from build123d import *

# Parameters (mm, degrees)
F1_DEPTH = 25
F2_R     = 8
F3_DEPTH = 25
F4_SIZE  = 5
F5_R     = 1.75
F6_DEPTH = 25


with BuildPart() as f1:
    # F0 (on Right) → F1 (new body)
    with BuildSketch(Plane.YZ):
        with BuildLine():
            Line((1.7320508076, 42.9015853287), (0, 41.9015853287))
            Line((0, 41.9015853287), (21, 5.5285183697))
            ThreePointArc((21, 5.5285183697), (22.8301270189, 3.6983913508), (25.3301270189, 3.0285183697))
            Line((25.3301270189, 3.0285183697), (72.3301270189, 3.0285183697))
            Line((72.3301270189, 3.0285183697), (72.3301270189, 5.0285183697))
            Line((72.3301270189, 5.0285183697), (25.3301270189, 5.0285183697))
            ThreePointArc((25.3301270189, 5.0285183697), (23.8301270189, 5.4304421584), (22.7320508076, 6.5285183697))
            Line((22.7320508076, 6.5285183697), (1.7320508076, 42.9015853287))
        make_face()
    extrude(amount=F1_DEPTH)

    # F2 (on face) → F3 (cut)
    with BuildSketch(Plane(origin=(0, 19.8759694843, 11.4753963322), x_dir=(-1, 0, 0), z_dir=(0, 0.8660254038, 0.5))):
        with Locations((-12.5, 24.2878373535)):
            Circle(F2_R)
    extrude(amount=-F3_DEPTH, mode=Mode.SUBTRACT)

    # F4
    f4_edges = [f1.edges().sort_by_distance(p)[0] for p in [
        (0, 0.866025, 42.401585),
        (25, 0.866025, 42.401585),
    ]]
    chamfer(f4_edges, length=F4_SIZE)

    # F5 (on face) → F6 (cut)
    with BuildSketch(Plane.XY.offset(5.0285183697)):
        with Locations((12.5, 63.3301270189)):
            Circle(F5_R)
        with Locations((12.5, 48.3301270189)):
            Circle(F5_R)
    extrude(amount=-F6_DEPTH, mode=Mode.SUBTRACT)


solid = f1.part
Build history of the part. All positions in model axes, mm. Round coordinates to 2 decimals unless told otherwise and drop trailing zeros. Loops run counter-clockwise (first coordinate to the right, second up) from the corner with the lowest first, then second, coordinate; pieces in that order, holes last. Notation, with made-up numbers: (12.25, 60) -> (63.25, 60) arc R19 ccw to (63.25, 65) -> close; hole circle Ø11 at (84.25, 65). An arc over 180 degrees is marked (long way). Answer in a Markdown table with one row per item.
Item 1: Saw through at B-B (y = 39). Write the cut outline in (x, z), and give its area (3 significant figures).
Answers below:
| item | result |
|---|---|
| outline | (0, 3.03) -> (25, 3.03) -> (25, 5.03) -> (0, 5.03) -> close |
| area | 50.0 mm² |
Item 2: Saw through at A-A (x = 12.5). Write the cut outline in (y, z).
Answers below:
| item | result |
|---|---|
| outline | (0, 41.9) -> (2, 38.44) -> (3.73, 39.44) -> (1.73, 42.9) -> close; (10, 24.58) -> (21, 5.53) arc R5 ccw to (25.33, 3.03) -> (46.58, 3.03) -> (46.58, 5.03) -> (25.33, 5.03) arc R3 cw to (22.73, 6.53) -> (11.73, 25.58) -> close; (50.08, 3.03) -> (61.58, 3.03) -> (61.58, 5.03) -> (50.08, 5.03) -> close; (65.08, 3.03) -> (72.33, 3.03) -> (72.33, 5.03) -> (65.08, 5.03) -> close |
Item 3: Pin check, flat tips, straight feed: pin 1 (8 mm diameter, centred on x = 11, z = 29.5, fed in from +Y); pin 2 (10 mm diameter, centred on x = 11.5, z = 8.5, fed in from -Y); pin 3 (6 mm diameter, centred on x = 5, z = 14.5, fed in from -Y). Stop position of each tip, or through.
Answers below:
| item | result |
|---|---|
| pin 1 | stops at y = 11.78 |
| pin 2 | stops at y = 16.4 |
| pin 3 | stops at y = 14.09 |
Item 4: Mould opens along X. For faces 1 (the cylindrical face through (12.272, 65.065, 4.043)), 2 (the flat face through (2.46, 2.15, 40.21)), 3 (the cylindrical face through (8.81, 10.43, 25.87)), 4 (the flat face through (10, 49, 5.029)) say: +X half, -X half, draft (parallel to the pull), parting line (faces both ways), or undercut.
Answers below:
| item | result |
|---|---|
| face 1 | undercut |
| face 2 | -X half |
| face 3 | undercut |
| face 4 | draft |
Item 5: Drill centre lines: L1, parallel to Y at x = 12.5, z = 3.6; L2, parallel to Y at x = 12.5, z = 4.65; L3, parallel to Z at x = 5.75, y = 37.5. Where is each one in solid material? Low to high. Write a range as [from, to].
Answers below:
| item | result |
|---|---|
| L1 | y = [23.01, 46.58], [50.08, 61.58], [65.08, 72.33] |
| L2 | y = [21.64, 46.58], [50.08, 61.58], [65.08, 72.33] |
| L3 | z = [3.03, 5.03] |
Item 6: Saw through at D-D (x = 23.5). Write the cut outline in (y, z).
Answers below:
| item | result |
|---|---|
| outline | (1.75, 38.87) -> (21, 5.53) arc R5 ccw to (25.33, 3.03) -> (72.33, 3.03) -> (72.33, 5.03) -> (25.33, 5.03) arc R3 cw to (22.73, 6.53) -> (3.48, 39.87) -> close |
Item 7: Saw through at C-C (z = 22.5). Write the cut outline in (x, y).
Answers below:
| item | result |
|---|---|
| outline | (0, 11.2) -> (25, 11.2) -> (25, 13.51) -> (0, 13.51) -> close |
